```python
from build123d import *

# Parameters (mm, degrees)
BOSS_EXTRUDE1_DEPTH    = 400
SKETCH2_R              = 3
SKETCH2_R_2            = 11.5
CUT_EXTRUDE1_DEPTH     = 10
CUT_EXTRUDE2_DEPTH     = 411.492681542
FILLET1_R              = 10
FILLET2_R              = 10
CONVERT_SOLID1_DEPTH   = 400
CONVERT_SOLID1_2_DEPTH = 400


# Read off the part's stored shape, not the designer's step: Convert-Solid1
with BuildPart() as part:
    # Sketch1 → Boss-Extrude1 (new body)
    with BuildSketch(Plane(origin=(0, 0, 0), x_dir=(0, 0, -1), z_dir=(1, 0, 0))):
        Polygon((-30.250452528, -29.403692131), (-40, 50), (30, 50), (30, 56), (-46.781766318, 56), (-36.205729437, -30.134908192), align=None)
    extrude(amount=BOSS_EXTRUDE1_DEPTH)

    # Sketch2 → Cut-Extrude1 (cut)
    with BuildSketch(Plane(origin=(0, -4.827047129, 39.313144045), x_dir=(1, 0, 0), z_dir=(0, -0.12186934340515194, 0.9925461516413215))):
        with Locations(Location((96, 36.283847636, 0), (0, 0, 270))):
            Circle(SKETCH2_R)
        with Locations(Location((294, 36.283847636, 0), (0, 0, 270))):
            Circle(SKETCH2_R)
        with Locations(Location((294, -13.716152364, 0), (0, 0, 270))):
            Circle(SKETCH2_R)
        with Locations(Location((60, 36.283847636, 0), (0, 0, 270))):
            Circle(SKETCH2_R_2)
        with Locations(Location((82.79, -13.716152364, 0), (0, 0, 270))):
            Circle(SKETCH2_R)
    extrude(amount=-CUT_EXTRUDE1_DEPTH, mode=Mode.SUBTRACT)

    # Sketch3 → Cut-Extrude2 (cut, through all)
    with BuildSketch(Plane(origin=(0, -4.827047129, 39.313144045), x_dir=(1, 0, 0), z_dir=(0, -0.12186934340515194, 0.9925461516413215))):
        Polygon((314, -25.497918682), (400, 39.502081318), (421.348881307, 33.662382961), (421.69701633, -53.203923072), (314, -56.960779507), align=None)
        Polygon((-35.970836278, 39.502081318), (0, 39.502081318), (62.79, -25.497918682), (64.049370498, -44.831722112), (-31.822947487, -47.152069291), align=None)
    extrude(amount=-CUT_EXTRUDE2_DEPTH, mode=Mode.SUBTRACT)

    # Fillet1
    fillet1_edges = [part.edges().sort_by_distance(p)[0] for p in [
        (400, 34.746199695, 41.149598304),
        (314, -29.769300162, 33.228090983),
        (0, 34.746199695, 41.149598304),
        (62.79, -29.769300162, 33.228090983),
    ]]
    fillet(fillet1_edges, radius=FILLET1_R)

    # Fillet2
    fillet2_edges = [part.edges().sort_by_distance(p)[0] for p in [
        (400, 53, -30),
        (0, 53, -30),
    ]]
    fillet(fillet2_edges, radius=FILLET2_R)

    # Convert-Solid1 outline → Convert-Solid1 (cut)
    with BuildSketch(Plane.YZ):
        with BuildLine():
            ThreePointArc((48.371288465, 45.845078322), (53.705816328, 44.188663392), (56, 39.095764491))
            Line((56, 39.095764491), (56, 46.781766318))
            Line((56, 46.781766318), (48.371288465, 45.845078322))
        make_face()
    extrude(amount=CONVERT_SOLID1_DEPTH, mode=Mode.SUBTRACT)

    # Convert-Solid1 2 outline → Convert-Solid1 2 (add)
    with BuildSketch(Plane.YZ):
        with BuildLine():
            ThreePointArc((49.102504525, 39.889801412), (49.730096039, 39.694929068), (50, 39.095764491))
            Line((50, 39.095764491), (50, 40))
            Line((50, 40), (49.102504525, 39.889801412))
        make_face()
    extrude(amount=CONVERT_SOLID1_2_DEPTH)


solid = part.part
```
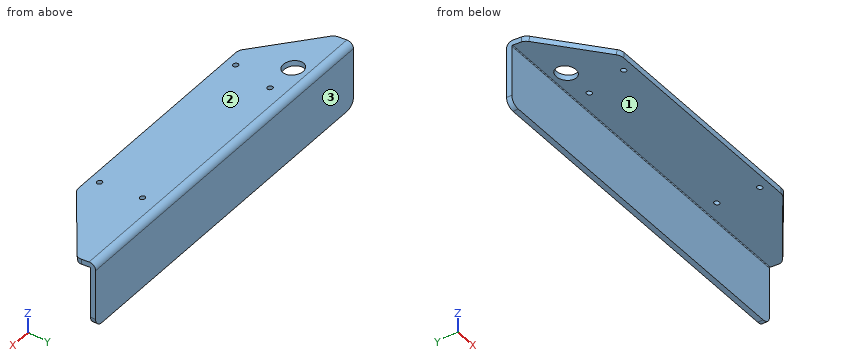
Input: part model. Units: mm. Frame: model coordinates. Face numbers are marked on the shaded views. Round coordinates to 2 decimals unless told otherwise and drop trailing zeros. Loops run counter-clockwise (first coordinate to the right, second up) from the corner with the lowest first, then second, coordinate; pieces in that order, holes last. Notation, with made-up numbers: (43, 74) - (66, 74) arc R22 ccw to (66, 110) - close; hole circle Ø4 at (22.5, -35.5). An arc over 180 degrees is marked (long way). One line per item, written item: value. Start each with the question number.
(1) Ray query, line 1 (X direction, y = -19, z = 37); line 2 (Y direction, x = 206, z = 18); line 3 (Z direction, x = 130, y = 29). Return the intervals inside material, ascending. Write a range as [from, to].
(2) Contact query for flat-ended pins moving along their axis: P1, Ø12, axis at y = 14.5, z = 34, coming from the -X side; P2, Ø2, axis at x = 339.5, y = 1, coming from the -Z side; P3, Ø10, axis at x = 94, y = 13, coming from the -Z side. Output: stop coordinate, or through.
(3) Section C-C, the plane y = -8. Return loops of the section in (x, z).
(4) Section A-A, the plane x = 220.5. Return loops of the section in (y, z).
(5) Section D-D, the plane x = 340. Return loops of the section in (y, z).
(6) Section B-B, the plane z = 0. Return loops of the section in (x, y).
(7) Draft query along Y for the marked faces 1, 2 and 3. Return one class per face: +Y half, -Y half, draft (parallel to the pull), parting line (faces both ways), or undercut.
Results below:
1. line 1: [52.02, 79.86], [85.72, 291.07], [296.93, 328.75]
1. line 2: [50, 56]
1. line 3: [37.42, 43.47]
2. P1: x = 14.68
2. P2: z = 33.86
2. P3: z = 34.84
3. outline: (41.25, 38.92) - (41.96, 32.88) - (342.53, 32.88) - (343.51, 38.92) - close
4. outline: (-30.13, 36.21) - (-29.4, 30.25) - (49.1, 39.89) arc R0.8 cw to (50, 39.1) - (50, -30) - (56, -30) - (56, 39.1) arc R6.8 ccw to (48.37, 45.85) - close
5. outline: (-10.63, 38.6) - (-9.9, 32.65) - (49.1, 39.89) arc R0.8 cw to (50, 39.1) - (50, -30) - (56, -30) - (56, 39.1) arc R6.8 ccw to (48.37, 45.85) - close
6. outline: (0, 50) - (400, 50) - (400, 56) - (0, 56) - close
7. face 1: undercut
7. face 2: -Y half
7. face 3: +Y half
